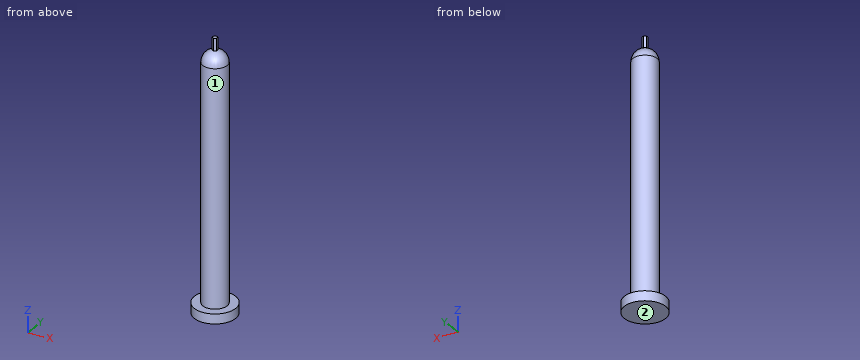
from build123d import *

# Parameters (mm, degrees)
F0_R     = 8.5
F1_DEPTH = 4
F2_R     = 5
F3_DEPTH = 100
F9_DEPTH = 5


with BuildPart() as f1:
    # F0 (on Top) → F1 (new body)
    with BuildSketch(Plane.XY):
        Circle(F0_R)
    extrude(amount=F1_DEPTH)

    # F2 (on Top) → F3 (join)
    with BuildSketch(Plane.XY):
        Circle(F2_R)
    extrude(amount=F3_DEPTH)

    # F4 (on Right) → F7 (revolve)
    with BuildSketch(Plane.YZ):
        with BuildLine():
            Line((0, 104.898979), (0, 100))
            Line((0, 100), (5, 100))
            ThreePointArc((5, 100), (3.872983, 103.162278), (1, 104.898979))
            Line((1, 104.898979), (0, 104.898979))
        make_face()
    revolve(axis=Axis((0, 0, 102.5), (0, 0, -1)))

    # F8 (on face) → F9 (join)
    with BuildSketch(Plane(origin=(0, 0, 104.898979), x_dir=(1, 0, 0), z_dir=(0, 0, -1))):
        Polygon((0.866025, -0.5), (0.866025, 0.5), (0, 1), (-0.866025, 0.5), (-0.866025, -0.5), (0, -1), align=None)
    extrude(amount=-F9_DEPTH)


solid = f1.part
Build history of the part. All positions in model axes, mm. Face numbers are marked on the shaded views. A direction names the side the tool comes from. Round coordinates to 2 decimals unless told otherwise and drop trailing zeros. Write each loop counter-clockwise with the first axis right and the second up, starting at its lowest first coordinate (ties: lowest second). Pieces come first, ordered by that corner, then holes. Notation, with made-up numbers: M 6.25,69 L 19.25,69 A32 ccw 19.25,108 Z; hole C 80,19 d1. An arc over 180 degrees is marked long. Answer as a JSON object with one key per item and string values. Group by question number.
(1) Which spindle directions (+Z, -Z, +X, -X, +Y, -Y) get a long thin tool onto all of the face, cutting with end or side? Do the marked faces 1 and 2. Say none if no direction does.
(2) Flat gauge pins, fed straight in: pin 1 (4 mm diameter, centred on y = -1.5, z = 12, fed in from -X); pin 2 (0.8 mm diameter, centred on y = 0, z = 107.5, fed in from +X); pin 3 (5 mm diameter, centred on x = -5.5, y = -7, fed in from +Z). Where does each tip first touch, or does it go through?
(3) Drill centre lines: L1, parallel to Z at x = 6.75, y = 2; L2, parallel to Y at x = -0.25, z = 17.5; L3, parallel to X at y = 0, z = 42. Where is each one in solid material? Low to high.
(4) Cut at A-A (z = 38.5). Give the cut face in (x, y), and give its area (3 significant figures).
(5) Cut at B-B (y = -6.75). Give the cut face in (x, z).
(6) Cut at C-C (x = -6). Give the cut face in (y, z), and give its area (3 significant figures).
Responses:
{
 "1": {"face 1": "+Z", "face 2": "-Z, +X, -X, +Y, -Y"},
 "2": {"pin 1": "stops at x = -5", "pin 2": "stops at x = 0.87", "pin 3": "stops at z = 4"},
 "3": {"L1": "z = 0 to 4", "L2": "y = -4.99 to 4.99", "L3": "x = -5 to 5"},
 "4": {"outline": "C 0,0 d10", "area": "78.5 mm2"},
 "5": {"outline": "M -5.17,0 L 5.17,0 L 5.17,4 L -5.17,4 Z"},
 "6": {"outline": "M -6.02,0 L 6.02,0 L 6.02,4 L -6.02,4 Z", "area": "48.2 mm2"}
}
